Can you work these out from the model? Positions are in its coordinate system, mm. A direction names the side the tool comes from. Round coordinates to 2 decimals unless told otherwise and drop trailing zeros. Loops run counter-clockwise (first coordinate to the right, second up) from the corner with the lowest first, then second, coordinate; pieces in that order, holes last. Notation, with made-up numbers: (75.5, -6) -> (96.5, -6) arc R18 ccw to (96.5, 3) -> close; hole circle Ø3 at (-4.75, 83). An arc over 180 degrees is marked (long way). Use a Markdown table: item, result.
from build123d import *

# Parameters (mm, degrees)
ESTRUSIONE_ESTRUSIONE1_DEPTH           = 5.09
FORO_SVASATO_PER_VITE_M3_1_D           = 3.4
FORO_SVASATO_PER_VITE_M3_1_CSINK_D     = 6.3
FORO_SVASATO_PER_VITE_M3_1_CSINK_ANGLE = 90
FORO_FILETTATO_M3X0_5_1_D              = 2.5
FORO_FILETTATO_M3X0_5_1_DEPTH          = 9
FORO_FILETTATO_M3X0_5_1_TIP            = 0.751075774
FORO_FILETTATO_M3X0_5_2_D              = 2.5
FORO_FILETTATO_M3X0_5_2_DEPTH          = 9
FORO_FILETTATO_M3X0_5_2_TIP            = 0.751075774
FORO_FILETTATO_M3X0_5_3_D              = 2.5
FORO_FILETTATO_M3X0_5_3_DEPTH          = 9
FORO_FILETTATO_M3X0_5_3_TIP            = 0.751075774
FORO_FILETTATO_M3X0_5_4_D              = 2.5


with BuildPart() as part:
    # Schizzo2 → Estrusione-Estrusione1 (new body)
    with BuildSketch(Plane.XY):
        with BuildLine():
            Line((13.408661509, 34.046761388), (25.008661509, 28.874777457))
            Line((25.008661509, 28.874777457), (25.008661509, 21.197917302))
            Line((25.008661509, 21.197917302), (28.539563234, 21.197917302))
            add(Edge.make_bspline(
                [(28.539563234, 21.197917302), (29.672665245, 21.054672347), (31.442336464, 20.883728728), (33.709967859, 19.337881701), (33.860174007, 17.780017142), (34.031169837, 17.055524547)],
                knots=[0, 0, 0, 0, 0.44666859, 0.69482561, 1, 1, 1, 1], degree=3))
            Line((34.031169837, 17.055524547), (34.031169837, 10.079137282))
            Line((34.031169837, 10.079137282), (39.054168668, 10.079137282))
            Line((39.054168668, 10.079137282), (39.054168668, 19.723110995))
            ThreePointArc((39.054168668, 19.723110995), (39.347061887, 20.430217776), (40.054168668, 20.723110995))
            Line((40.054168668, 20.723110995), (43.156897639, 20.723110995))
            ThreePointArc((43.156897639, 20.723110995), (43.86400442, 20.430217776), (44.156897639, 19.723110995))
            Line((44.156897639, 19.723110995), (44.156897639, 10.059204747))
            Line((44.156897639, 10.059204747), (49.080233794, 10.059204747))
            Line((49.080233794, 10.059204747), (49.080233794, 17.055524547))
            add(Edge.make_bspline(
                [(49.080233794, 17.055524547), (48.967324691, 18.346340588), (50.999627836, 20.921028345), (54.113128084, 21.035559742), (55.71736734, 21.197917302)],
                knots=[0, 0, 0, 0, 0.423714054, 1, 1, 1, 1], degree=3))
            Line((55.71736734, 21.197917302), (63.258661509, 21.197917302))
            Line((63.258661509, 21.197917302), (63.258661509, 28.539967348))
            add(Edge.make_bspline(
                [(63.258661509, 28.539967348), (62.239722551, 28.759416988), (61.253896648, 30.182238688), (61.448846017, 32.629580504), (62.536492347, 33.654111413), (63.258661509, 33.978194592)],
                knots=[0, 0, 0, 0, 0.415878439, 0.65656192, 1, 1, 1, 1], degree=3))
            Line((63.258661509, 33.978194592), (63.258661509, 39.997917302))
            Line((63.258661509, 39.997917302), (59.258661509, 39.997917302))
            ThreePointArc((59.258661509, 39.997917302), (41.848661509, 35.197917302), (24.438661509, 39.997917302))
            Line((24.438661509, 39.997917302), (13.408661509, 39.997917302))
            Line((13.408661509, 39.997917302), (13.408661509, 34.046761388))
        make_face()
    extrude(amount=ESTRUSIONE_ESTRUSIONE1_DEPTH)

    # Foro svasato per Vite M3-1 (through all)
    with Locations(Plane(origin=(0, 0, 0), x_dir=(-1, 0, 0), z_dir=(0, 0, -1))):
        with Locations((-48.605533153, 32.579137282), (-34.605533153, 32.579137282)):
            CounterSinkHole(FORO_SVASATO_PER_VITE_M3_1_D / 2, FORO_SVASATO_PER_VITE_M3_1_CSINK_D / 2, counter_sink_angle=FORO_SVASATO_PER_VITE_M3_1_CSINK_ANGLE)

    # Foro filettato M3x0.5-1
    with Locations(Plane(origin=(63.258661509, 0, 0), x_dir=(0, 0, -1), z_dir=(1, 0, 0))):
        with Locations((-2.545, 36.847917302), (-2.545, 24.347917302)):
            Hole(FORO_FILETTATO_M3X0_5_1_D / 2, depth=FORO_FILETTATO_M3X0_5_1_DEPTH)
            with Locations((0, 0, -(FORO_FILETTATO_M3X0_5_1_DEPTH + FORO_FILETTATO_M3X0_5_1_TIP / 2))):  # 118° drill point
                Cone(0, FORO_FILETTATO_M3X0_5_1_D / 2, FORO_FILETTATO_M3X0_5_1_TIP, mode=Mode.SUBTRACT)

    # Foro filettato M3x0.5-2
    with Locations(Plane.ZY.offset(-13.408661509)):
        with Locations((2.545, 36.847917302)):
            Hole(FORO_FILETTATO_M3X0_5_2_D / 2, depth=FORO_FILETTATO_M3X0_5_2_DEPTH)
            with Locations((0, 0, -(FORO_FILETTATO_M3X0_5_2_DEPTH + FORO_FILETTATO_M3X0_5_2_TIP / 2))):  # 118° drill point
                Cone(0, FORO_FILETTATO_M3X0_5_2_D / 2, FORO_FILETTATO_M3X0_5_2_TIP, mode=Mode.SUBTRACT)

    # Foro filettato M3x0.5-3
    with Locations(Plane.ZY.offset(-25.008661509)):
        with Locations((2.545, 24.347917302)):
            Hole(FORO_FILETTATO_M3X0_5_3_D / 2, depth=FORO_FILETTATO_M3X0_5_3_DEPTH)
            with Locations((0, 0, -(FORO_FILETTATO_M3X0_5_3_DEPTH + FORO_FILETTATO_M3X0_5_3_TIP / 2))):  # 118° drill point
                Cone(0, FORO_FILETTATO_M3X0_5_3_D / 2, FORO_FILETTATO_M3X0_5_3_TIP, mode=Mode.SUBTRACT)

    # Foro filettato M3x0.5-4 (through all)
    with Locations(Plane(origin=(49.080233794, 0, 0), x_dir=(0, 0, -1), z_dir=(1, 0, 0))):
        with Locations((-2.545, 12.604204747)):
            Hole(FORO_FILETTATO_M3X0_5_4_D / 2)


solid = part.part
1. I want a section at D-D (x = 26). Please give me the cut outline in (y, z) (3 decimals).
Answer sheet:
| item | result |
|---|---|
| outline | (21.198, 0) -> (39.121, 0) -> (39.121, 5.09) -> (21.198, 5.09) -> close; hole circle Ø2.5 at (24.348, 2.545) |
2. If we mould it in two halves opening along X, with no side actions, what happens to faces 4 (the flat face through (44.157, 15, 3)), 5 (the flat face through (13.409, 38.4, 2.5)), 6 (the cylindrical face through (58.7, 35.63, 2.27))? For each: +X half, -X half, draft (parallel to the pull), parting line (faces both ways), or undercut.
Answer sheet:
| item | result |
|---|---|
| face 4 | undercut |
| face 5 | -X half |
| face 6 | draft |
3. I need wall thicknesses on line 1 (Y direction, x = 35.5, z = 2.4); line 2 (X direction, y = 33.5, z = 4.2); line 3 (X direction, y = 12.75, z = 1.2). Which ranges of each line are inside material? Lowest first, please.
Answer sheet:
| item | result |
|---|---|
| line 1 | y = 10.08 to 11.36, 13.85 to 31.13, 34.02 to 35.8 |
| line 2 | x = 14.63 to 33.18, 36.03 to 47.18, 50.03 to 62.49 |
| line 3 | x = 34.03 to 39.05, 44.16 to 49.08 |
4. Will these pins go through, and if not, where does the flat tip stop? pin 1 Ø2 at (x, z) = (30.5, 3) entering from -Y; pin 2 Ø2.5 at (x, z) = (60.5, 2.5) entering from -Y; pin 3 Ø3 at (y, z) = (36.85, 2.54) entering from +X; pin 4 Ø2.5 at (x, z) = (41.5, 3) entering from -Y.
Answer sheet:
| item | result |
|---|---|
| pin 1 | stops at y = 20.61 |
| pin 2 | stops at y = 21.2 |
| pin 3 | stops at x = 63.26 |
| pin 4 | stops at y = 20.72 |
5. I want a section at A-A (y = 13.25). Please give me the cut outline in (x, z), plus the area to 3 significant figures.
Answer sheet:
| item | result |
|---|---|
| outline | (34.03, 0) -> (39.05, 0) -> (39.05, 1.47) -> (34.03, 1.47) -> close; (34.03, 3.62) -> (39.05, 3.62) -> (39.05, 5.09) -> (34.03, 5.09) -> close; (44.16, 0) -> (49.08, 0) -> (49.08, 1.47) -> (44.16, 1.47) -> close; (44.16, 3.62) -> (49.08, 3.62) -> (49.08, 5.09) -> (44.16, 5.09) -> close |
| area | 29.3 mm² |
6. I want a section at B-B (x = 58.5). Please give me the cut outline in (y, z) (3 decimals), plus the area to 3 significant figures.
Answer sheet:
| item | result |
|---|---|
| outline | (21.198, 0) -> (39.558, 0) -> (39.558, 5.09) -> (21.198, 5.09) -> close; hole circle Ø2.5 at (24.348, 2.545); hole circle Ø2.5 at (36.848, 2.545) |
| area | 83.6 mm² |
7. I want a section at C-C (z = 3.1). State how many separate pieces and enclosed holes the cut face has, plus the area to 3 significant figures.
Answer sheet:
| item | result |
|---|---|
| separate pieces | 4 |
| enclosed holes | 2 |
| area | 698 mm² |
8. Which directions (+Z, -Z, +X, -X, +Y, -Y) give clear straight access to the entire face, cutting with the end or side of a thin tool? Please do faces 1 (the cylindrical face through (17.972, 38.087, 2.708)), 2 (the flat face through (25.009, 26, 3)), 3 (the flat face through (42, 20.723, 3)).
Answer sheet:
| item | result |
|---|---|
| face 1 | -X |
| face 2 | +Z, -Z, -X, -Y |
| face 3 | +Z, -Z, -Y |
